Verification items for the finished model (mm, model axes). Face numbers are marked on the shaded views. Coordinates: 2 decimals unless noted, no trailing zeros. Loops run counter-clockwise (first coordinate to the right, second up) from the corner with the lowest first, then second, coordinate; pieces in that order, holes last.
Q1. Sectioned sample at C-C (x = -58). Enter the section's corners in (y, z), then the cut area to 3 significant figures.
Q2. Sectioned sample at B-B (z = 4). Enter the section's corners in (x, y), then the cut area to 3 significant figures.
Q3. Material ranges on probe 1 along Y at (x, z) = (-49.75, 0.75); probe 2 along Y at (x, z) = (71.5, 0.25); probe 3 along Y at (x, z) = (-26, 14), recorded low to high.
Q4. Go/stop test with flat-tipped pins: P1, Ø19, axis at x = 8.5, y = 8.5, coming from the +Z side; P2, Ø1.5, axis at x = -55, y = 2.5, coming from the +Z side; P3, Ø3, axis at y = 18, z = 18.5, coming from the -X side; P4, Ø8, axis at y = -1, z = 13.5, coming from the +X side. Record where each tip stops, or that it passes through.
Q5. Sectioned sample at A-A (x = -81.25). Enter the section's corners in (y, z).
Q6. Mould release check, pull along Y, two halves, no side actions. Record for the marked faces 1, 2 and 3: +Y half, -Y half, draft (parallel to the pull), parting line (faces both ways), or undercut.
Q7. Sectioned sample at D-D (x = 36.5). Enter the section's corners in (y, z).
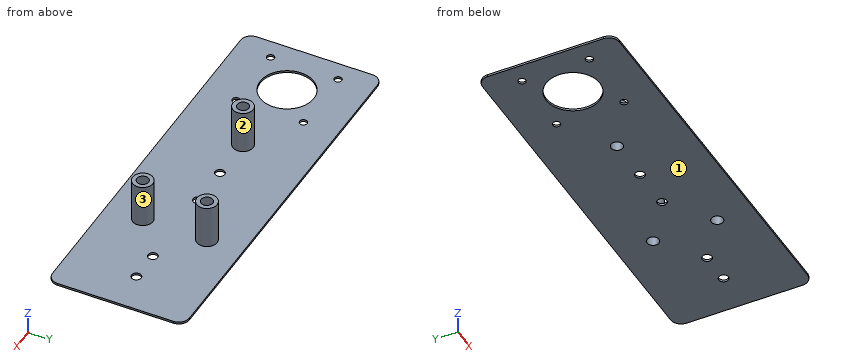
```python
from build123d import *

# Parameters (mm, degrees)
BOSS_EXTRUDE1_DEPTH = 37
SKETCH2_R           = 1.75
SKETCH2_R_2         = 12.5
SKETCH2_R_3         = 2.75
SKETCH2_R_4         = 2.25
CUT_EXTRUDE1_DEPTH  = 38
SKETCH5_R           = 2.25
CUT_EXTRUDE2_DEPTH  = 38
CUT_EXTRUDE3_DEPTH  = 36
SKETCH7_R           = 4.75
BOSS_EXTRUDE2_DEPTH = 20.5
SKETCH10_W          = 40
SKETCH10_H          = 64
CUT_EXTRUDE4_DEPTH  = 36
SKETCH11_R          = 2.75
CUT_EXTRUDE5_DEPTH  = 22.5
SKETCH12_W          = 15
SKETCH12_H          = 10
SKETCH12_W_2        = 20
SKETCH12_W_3        = 10
BOSS_EXTRUDE3_DEPTH = 36
CUT_EXTRUDE6_DEPTH  = 33
CUT_EXTRUDE8_DEPTH  = 15
CUT_EXTRUDE9_DEPTH  = 15
CUT_EXTRUDE10_DEPTH = 10
CUT_EXTRUDE11_DEPTH = 10
SKETCH20_W          = 6
SKETCH20_H          = 15
CUT_EXTRUDE12_DEPTH = 3
SKETCH21_W          = 76
SKETCH21_H          = 64
SKETCH21_W_2        = 9.5
SKETCH21_H_2        = 9.5
SKETCH21_W_3        = 65
CUT_EXTRUDE13_DEPTH = 36


with BuildPart() as part:
    # Sketch1 → Boss-Extrude1 (new body)
    with BuildSketch(Plane.XY):
        with BuildLine():
            Line((-85.5, 32), (85.5, 32))
            ThreePointArc((85.5, 32), (89.035533906, 30.535533906), (90.5, 27))
            Line((90.5, 27), (90.5, -27))
            ThreePointArc((90.5, -27), (89.035533906, -30.535533906), (85.5, -32))
            Line((85.5, -32), (-85.5, -32))
            ThreePointArc((-85.5, -32), (-89.035533906, -30.535533906), (-90.5, -27))
            Line((-90.5, -27), (-90.5, 27))
            ThreePointArc((-90.5, 27), (-89.035533906, 30.535533906), (-85.5, 32))
        make_face()
    extrude(amount=BOSS_EXTRUDE1_DEPTH)

    # Sketch2 → Cut-Extrude1 (cut, through all)
    with BuildSketch(Plane.XY.offset(37)):
        with Locations((-81.25, 15.75)):
            Circle(SKETCH2_R)
        with Locations((-49.75, 15.75)):
            Circle(SKETCH2_R)
        with Locations((-81.25, -15.75)):
            Circle(SKETCH2_R)
        with Locations((-49.75, -15.75)):
            Circle(SKETCH2_R)
        with Locations((-65.5, 0)):
            Circle(SKETCH2_R_2)
        with Locations((36.5, 15)):
            Circle(SKETCH2_R_3)
        with Locations((36.5, -15)):
            Circle(SKETCH2_R_3)
        with Locations((-25.5, 0)):
            Circle(SKETCH2_R_3)
        with Locations((56.5, 0)):
            Circle(SKETCH2_R_4)
        with Locations((71.5, 0)):
            Circle(SKETCH2_R_4)
    extrude(amount=-CUT_EXTRUDE1_DEPTH, mode=Mode.SUBTRACT)

    # Sketch5 → Cut-Extrude2 (cut, through all)
    with BuildSketch(Plane.XY.offset(37)):
        with Locations((-4.5, 0)):
            Circle(SKETCH5_R)
        with Locations((15.5, 0)):
            Circle(SKETCH5_R)
    extrude(amount=-CUT_EXTRUDE2_DEPTH, mode=Mode.SUBTRACT)

    # Sketch6 → Cut-Extrude3 (cut)
    with BuildSketch(Plane.XY.offset(37)):
        with BuildLine():
            Line((-85.5, -29), (85.5, -29))
            ThreePointArc((85.5, -29), (86.914213562, -28.414213562), (87.5, -27))
            Line((87.5, -27), (87.5, 27))
            ThreePointArc((87.5, 27), (86.914213562, 28.414213562), (85.5, 29))
            Line((85.5, 29), (-85.5, 29))
            ThreePointArc((-85.5, 29), (-86.914213562, 28.414213562), (-87.5, 27))
            Line((-87.5, 27), (-87.5, -27))
            ThreePointArc((-87.5, -27), (-86.914213562, -28.414213562), (-85.5, -29))
        make_face()
    extrude(amount=-CUT_EXTRUDE3_DEPTH, mode=Mode.SUBTRACT)

    # Sketch7 → Boss-Extrude2 (add)
    with BuildSketch(Plane.XY.offset(1)):
        with Locations((-25.5, 0)):
            Circle(SKETCH7_R)
        with Locations((36.5, -15)):
            Circle(SKETCH7_R)
        with Locations((36.5, 15)):
            Circle(SKETCH7_R)
    extrude(amount=BOSS_EXTRUDE2_DEPTH)

    # Sketch10 → Cut-Extrude4 (cut)
    with BuildSketch(Plane.XY.offset(37)):
        with Locations((5.5, 0)):
            Rectangle(SKETCH10_W, SKETCH10_H)
    extrude(amount=-CUT_EXTRUDE4_DEPTH, mode=Mode.SUBTRACT)

    # Sketch11 → Cut-Extrude5 (cut, through all)
    with BuildSketch(Plane.XY.offset(21.5)):
        with Locations((36.5, -15)):
            Circle(SKETCH11_R)
        with Locations((-25.5, 0)):
            Circle(SKETCH11_R)
        with Locations((36.5, 15)):
            Circle(SKETCH11_R)
    extrude(amount=-CUT_EXTRUDE5_DEPTH, mode=Mode.SUBTRACT)

    # Sketch12 → Boss-Extrude3 (add, through all)
    with BuildSketch(Plane.XY.offset(1)):
        with Locations((75, -24)):
            Rectangle(SKETCH12_W, SKETCH12_H)
        with Locations((75, 24)):
            Rectangle(SKETCH12_W, SKETCH12_H)
        with Locations((77.5, -11)):
            Rectangle(SKETCH12_W_2, SKETCH12_H)
        with Locations((77.5, 11)):
            Rectangle(SKETCH12_W_2, SKETCH12_H)
        with Locations((-37.5, -24)):
            Rectangle(SKETCH12_W_3, SKETCH12_H)
        with Locations((-37.5, 24)):
            Rectangle(SKETCH12_W_3, SKETCH12_H)
    extrude(amount=BOSS_EXTRUDE3_DEPTH)

    # Sketch14 → Cut-Extrude6 (cut)
    with BuildSketch(Plane.XZ.offset(16)):
        Polygon((87.5, 37), (67.5, 37), (67.5, 3), align=None)
    extrude(amount=-CUT_EXTRUDE6_DEPTH, mode=Mode.SUBTRACT)

    # Sketch16 → Cut-Extrude8 (cut)
    with BuildSketch(Plane(origin=(82.5, 0, 0), x_dir=(0, 0, -1), z_dir=(1, 0, 0))):
        Polygon((-37, -19), (-3, -19), (-37, -29), align=None)
    extrude(amount=-CUT_EXTRUDE8_DEPTH, mode=Mode.SUBTRACT)

    # Sketch17 → Cut-Extrude9 (cut)
    with BuildSketch(Plane.ZY.offset(-67.5)):
        Polygon((37, 19), (1, 19), (37, 29), align=None)
    extrude(amount=-CUT_EXTRUDE9_DEPTH, mode=Mode.SUBTRACT)

    # Sketch18 → Cut-Extrude10 (cut)
    with BuildSketch(Plane(origin=(-32.5, 0, 0), x_dir=(0, 0, -1), z_dir=(1, 0, 0))):
        Polygon((-37, -29), (-37, -19), (-1, -19), align=None)
    extrude(amount=-CUT_EXTRUDE10_DEPTH, mode=Mode.SUBTRACT)

    # Sketch19 → Cut-Extrude11 (cut)
    with BuildSketch(Plane(origin=(-32.5, 0, 0), x_dir=(0, 0, -1), z_dir=(1, 0, 0))):
        Polygon((-37, 29), (-1, 19), (-37, 19), align=None)
    extrude(amount=-CUT_EXTRUDE11_DEPTH, mode=Mode.SUBTRACT)

    # Sketch20 → Cut-Extrude12 (cut)
    with BuildSketch(Plane.ZY.offset(90.5)):
        with Locations((30, 0)):
            Rectangle(SKETCH20_W, SKETCH20_H)
    extrude(amount=-CUT_EXTRUDE12_DEPTH, mode=Mode.SUBTRACT)

    # Sketch21 → Cut-Extrude13 (cut)
    with BuildSketch(Plane.XY.offset(37)):
        with Locations((-52.5, 0)):
            Rectangle(SKETCH21_W, SKETCH21_H)
        with Locations((-25.5, 0)):
            Rectangle(SKETCH21_W_2, SKETCH21_H_2, mode=Mode.SUBTRACT)
        with Locations((58, 0)):
            Rectangle(SKETCH21_W_3, SKETCH21_H)
        with Locations((36.5, -15)):
            Rectangle(SKETCH21_W_2, SKETCH21_H_2, mode=Mode.SUBTRACT)
        with Locations((36.5, 15)):
            Rectangle(SKETCH21_W_2, SKETCH21_H_2, mode=Mode.SUBTRACT)
    extrude(amount=-CUT_EXTRUDE13_DEPTH, mode=Mode.SUBTRACT)


solid = part.part
```
Geometry check:
1. outline: (-32, 0) - (-10, 0) - (-10, 1) - (-32, 1) - close; (10, 0) - (32, 0) - (32, 1) - (10, 1) - close
1. area: 44.0 mm2
2. outline: circle Ø9.5 at (-25.5, 0); circle Ø9.5 at (36.5, -15); circle Ø9.5 at (36.5, 15); hole circle Ø5.5 at (-25.5, 0); hole circle Ø5.5 at (36.5, -15); hole circle Ø5.5 at (36.5, 15)
2. area: 141 mm2
3. probe 1: y = -32 to -17.5, -14 to 14, 17.5 to 32
3. probe 2: y = -32 to -2.25, 2.25 to 32
3. probe 3: y = -4.72 to -2.7, 2.7 to 4.72
4. P1: stops at z = 1
4. P2: passes through
4. P3: stops at x = 31.99
4. P4: stops at x = -20.75
5. outline: (-32, 0) - (-17.5, 0) - (-17.5, 1) - (-32, 1) - close; (-14, 0) - (14, 0) - (14, 1) - (-14, 1) - close; (17.5, 0) - (32, 0) - (32, 1) - (17.5, 1) - close
6. face 1: draft
6. face 2: parting line
6. face 3: undercut
7. outline: (-32, 0) - (-17.75, 0) - (-17.75, 21.5) - (-19.75, 21.5) - (-19.75, 1) - (-32, 1) - close; (-12.25, 0) - (12.25, 0) - (12.25, 21.5) - (10.25, 21.5) - (10.25, 1) - (-10.25, 1) - (-10.25, 21.5) - (-12.25, 21.5) - close; (17.75, 0) - (32, 0) - (32, 1) - (19.75, 1) - (19.75, 21.5) - (17.75, 21.5) - close
